Part print with two shaded views. Sizes in mm from the minimum x, y, z corner. Round coordinates to 2 decimals unless told otherwise and drop trailing zeros. Write each loop counter-clockwise with the first axis right and the second up, starting at its lowest first coordinate (ties: lowest second). Pieces come first, ordered by that corner, then holes. Notation, with made-up numbers: (46, 5) -> (97, 5) arc R19 ccw to (97, 32) -> close; hole circle Ø11 at (45.5, 63). An arc over 180 degrees is marked (long way). Answer in a Markdown table with one row per item. Add a question column.
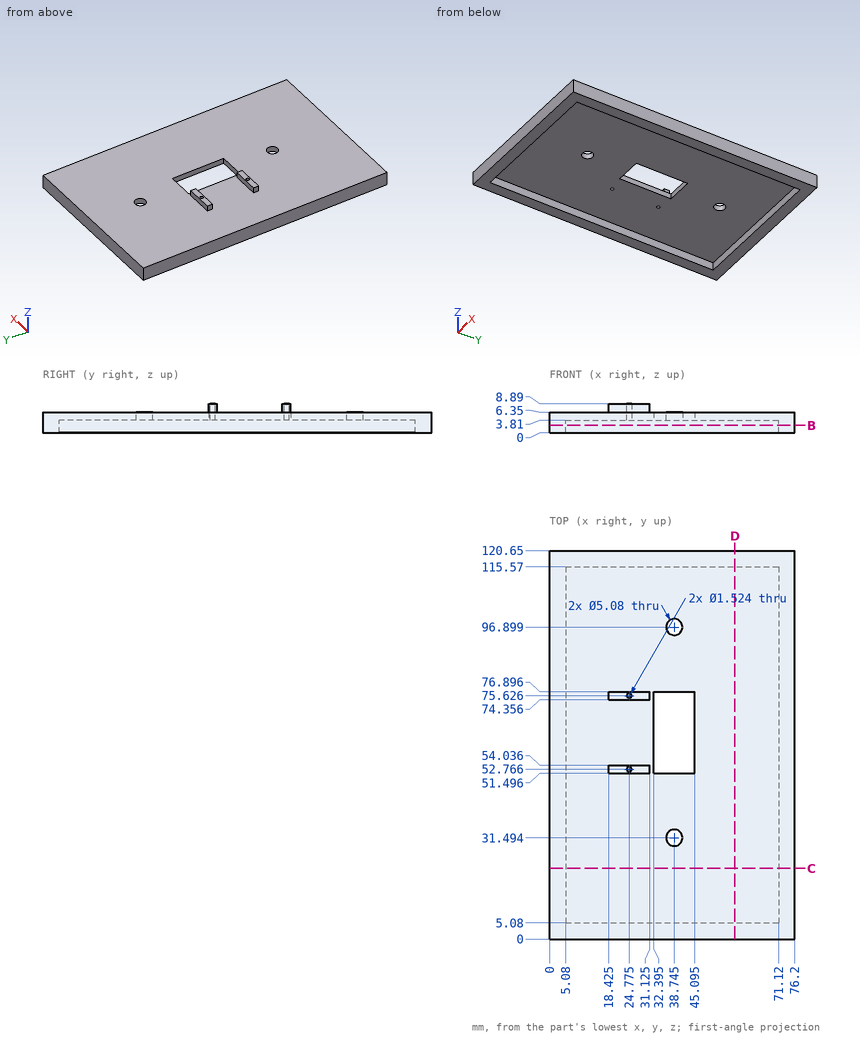
Item 1: Saw through at B-B on z = 2.25. Give the cut face in (x, y), then the cut area to 3 significant figures.
Item 2: Saw through at C-C on y = 22. Give the cut face in (x, z).
Item 3: Saw through at D-D on x = 57.5. Give the cut face in (y, z), then the cut area to 3 significant figures.
Item 4: Drill centre lines: probe 1 along X at (y, z) = (37.5, 1); probe 2 along Y at (x, z) = (9.5, 2.75); probe 3 along X at (y, z) = (64, 4.5) (1 decimal). Where is each one in solid material? Low to high.
Item 5: Pin check, flat tips, straight feed: pin 1 (6 mm diameter, centred on x = 38.74, y = 31.49, fed in from -Z); pin 2 (3 mm diameter, centred on x = 41.5, z = 5, fed in from -Y); pin 3 (1.3 mm diameter, centred on x = 24.5, z = 8, fed in from +Y); pin 4 (12 mm diameter, centred on x = 22.5, y = 64.5, fed in from +Z). Stop position of each tip, or through.
Recorded:
| question | item | result |
|---|---|---|
| 1 | outline | (0, 0) -> (76.2, 0) -> (76.2, 120.65) -> (0, 120.65) -> close; hole (5.08, 5.08) -> (71.12, 5.08) -> (71.12, 115.57) -> (5.08, 115.57) -> close |
| 1 | area | 1,900 mm2 |
| 2 | outline | (0, 0) -> (5.08, 0) -> (5.08, 3.81) -> (71.12, 3.81) -> (71.12, 0) -> (76.2, 0) -> (76.2, 6.35) -> (0, 6.35) -> close |
| 3 | outline | (0, 0) -> (5.08, 0) -> (5.08, 3.81) -> (115.57, 3.81) -> (115.57, 0) -> (120.65, 0) -> (120.65, 6.35) -> (0, 6.35) -> close |
| 3 | area | 345 mm2 |
| 4 | probe 1 | 0 to 5.08, 71.12 to 76.2 |
| 4 | probe 2 | 0 to 5.08, 115.57 to 120.65 |
| 4 | probe 3 | 0 to 32.4, 45.1 to 76.2 |
| 5 | pin 1 | z = 3.81 |
| 5 | pin 2 | y = 0 |
| 5 | pin 3 | y = 76.9 |
| 5 | pin 4 | z = 6.35 |
